```python
from build123d import *

# Parameters (mm, degrees)
F0_W     = 300
F0_H     = 5
F1_DEPTH = 150
F2_R     = 4
F3_DEPTH = 3


with BuildPart() as f1:
    # F0 (on Front) → F1 (new body, symmetric)
    with BuildSketch(Plane.XZ):
        Rectangle(F0_W, F0_H)
    extrude(amount=F1_DEPTH, both=True)

    # F2 (on Top) → F3 (cut, symmetric)
    with BuildSketch(Plane.XY):
        with Locations((138, -138)):
            Circle(F2_R)
        with Locations((-138, -138)):
            Circle(F2_R)
        with Locations((-138, 138)):
            Circle(F2_R)
        with Locations((138, 138)):
            Circle(F2_R)
    extrude(amount=F3_DEPTH, both=True, mode=Mode.SUBTRACT)


solid = f1.part
```
The model under review builds one solid part; all positions refer to its coordinate system, in mm. Round coordinates to 2 decimals unless told otherwise and drop trailing zeros. Loops run counter-clockwise (first coordinate to the right, second up) from the corner with the lowest first, then second, coordinate; pieces in that order, holes last. Notation, with made-up numbers: (85, 69) -> (110, 69) arc R12 cw to (110, 78) -> close; hole circle Ø8 at (-18, 88). An arc over 180 degrees is marked (long way). Answer as a JSON object with one key per item and string values. Group by question number.
1) For line 1 (Y direction, x = 138, z = 0.5), list the stretches that pass through material, from the lowest coordinate up. Write a range as [from, to].
2) Mouldability with a two-part tool opening along Y and no side actions: class faces 1 (the face through (-135.85, -134.627, 0.035)), 2 (the face through (-2, -2, 2.5)) as released by +Y, released by -Y, zero draft, split by the parting line, or undercut.
3) We need section A-A on x = 138. Write out the cut boundary in (y, z).
Result set:
{
 "1": {"line 1": "[-150, -142], [-134, 134], [142, 150]"},
 "2": {"face 1": "undercut", "face 2": "zero draft"},
 "3": {"outline": "(-150, -2.5) -> (-142, -2.5) -> (-142, 2.5) -> (-150, 2.5) -> close; (-134, -2.5) -> (134, -2.5) -> (134, 2.5) -> (-134, 2.5) -> close; (142, -2.5) -> (150, -2.5) -> (150, 2.5) -> (142, 2.5) -> close"}
}
